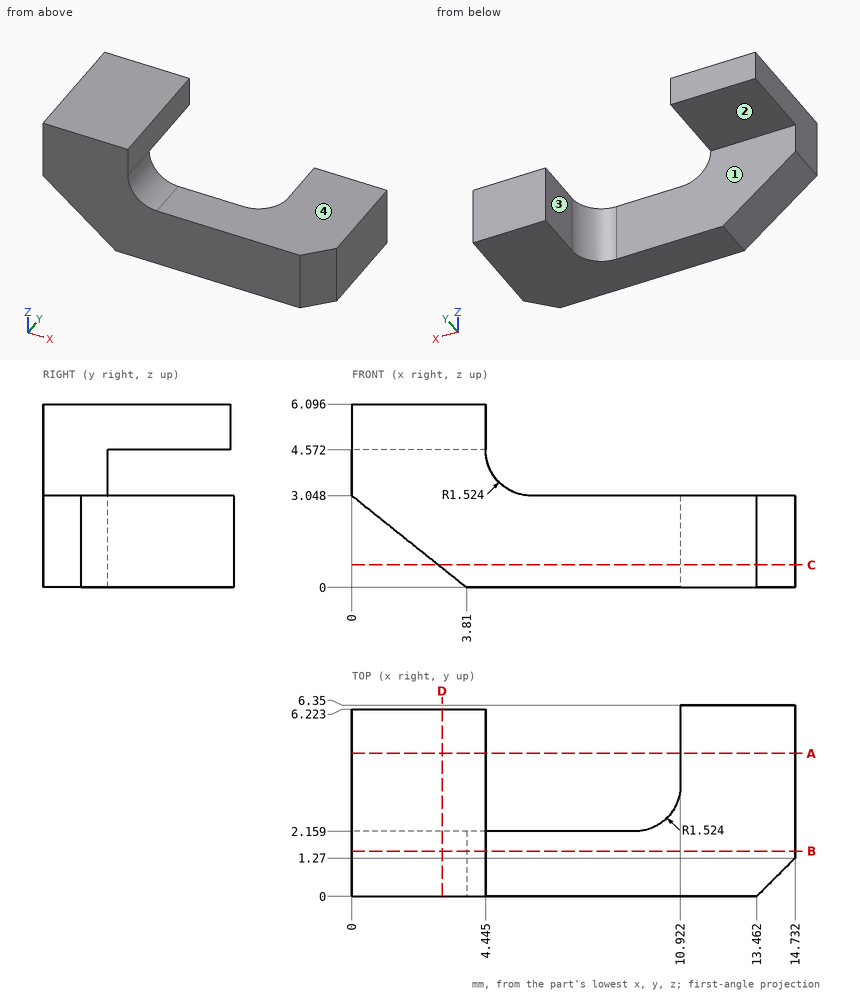
For this review, use the dimensioned drawing (mm, ordinates from the lowest corner) and the shaded views. A direction names the side the tool comes from. Round coordinates to 2 decimals unless told otherwise and drop trailing zeros. Loops run counter-clockwise (first coordinate to the right, second up) from the corner with the lowest first, then second, coordinate; pieces in that order, holes last. Notation, with made-up numbers: M -21,12.25 L -2,12.25 A16 cw -2,16.25 Z; hole C 70,69.5 d9. An arc over 180 degrees is marked long. Answer as CSV lines item,"result".
1. We need section C-C (z = 0.75). Give the boundary of the cut face in (x, y).
Outcome:
outline,"M 2.87,0 L 13.46,0 L 14.73,1.27 L 14.73,6.35 L 10.92,6.35 L 10.92,3.68 A1.52 cw 9.4,2.16 L 2.87,2.16 Z"
2. We need section B-B (y = 1.5). Give the boundary of the cut face in (x, z) (3 decimals), plus the area to 3 significant figures.
Outcome:
outline,"M 0,3.048 L 3.81,0 L 14.732,0 L 14.732,3.048 L 5.969,3.048 A1.524 cw 4.445,4.572 L 4.445,6.096 L 0,6.096 Z"
area,"53.1 mm2"
3. To check wall thickness, follow L1, parallel to Y at x = 6, z = 2.5; L2, parallel to X at y = 5, z = 2.25; L3, parallel to Z at x = 13.5, y = 3.5. State the ranges of each line that lie inside material, in increasing order. Write a range as [from, to].
Outcome:
L1,"y = [0, 2.16]"
L2,"x = [10.92, 14.73]"
L3,"z = [0, 3.05]"
4. For the marked faces 1, 2, 3 and 4, list the 3-axis set-ups (+Z, -Z, +X, -X, +Y, -Y) from which the entire face can be reached by the end or side of a thin tool; tool diameter is ignored.
Outcome:
face 1,"-Z, -X, +Y"
face 2,"-Z, +X, -X, +Y"
face 3,"+Z, -Z, -X, +Y"
face 4,"+Z, +X, +Y, -Y"
5. We need section D-D (x = 3). Give the boundary of the cut face in (y, z), plus the area to 3 significant figures.
Outcome:
outline,"M 0,0.65 L 2.16,0.65 L 2.16,4.57 L 6.22,4.57 L 6.22,6.1 L 0,6.1 Z"
area,"18.0 mm2"
6. We need section A-A (y = 4.75). Give the boundary of the cut face in (x, z) (3 decimals), plus the area to 3 significant figures.
Outcome:
outline,"M 0,4.572 L 4.445,4.572 L 4.445,6.096 L 0,6.096 Z; M 10.922,0 L 14.732,0 L 14.732,3.048 L 10.922,3.048 Z"
area,"18.4 mm2"
7. Insertion check: pin 1 Ø0.5 at (y, z) = (3, 5) entering from +X (3 decimals); pin 2 Ø1 at (x, z) = (7.5, 1.5) entering from +Y; pin 3 Ø1.5 at (x, y) = (7, 1) entering from +Z. Each pin has a flat end and moves straight along its axis. Give the tip position at first contact, or say it passes through.
Outcome:
pin 1,"stops at x = 4.445"
pin 2,"stops at y = 2.16"
pin 3,"stops at z = 3.05"
